Can you work these out from the model? Positions are in its coordinate system, mm. A direction names the side the tool comes from. Coordinates: 2 decimals unless noted, no trailing zeros. Order: outer loops, then holes, each group sorted by start corner. A loop starts at its lowest first (then second) coordinate and runs counter-clockwise, first axis right, second up. Notation, with made-up numbers: (5, -16.5) -> (40, -16.5) arc R18 ccw to (40, -12.5) -> close; hole circle Ø2 at (-29, 74). An arc over 180 degrees is marked (long way). Use a Markdown table: item, result. Add a question column.
1. For pin 1 Ø3.5 at (x, z) = (22.5, 19.5) entering from +Y; pin 2 Ø1.1 at (y, z) = (23, 19.5) entering from -X; pin 3 Ø4 at (x, z) = (18, 23) entering from +Y; pin 4 Ø6.5 at (y, z) = (-14.5, 16) entering from -X, each with a flat end and sliding along its axis, tell me the tip position at first contact or that it passes through.
2. If I drill on line 1 along X through (y, z) = (-5, 29.5); line 2 along Y through (x, z) = (19, 17), over which ranges is the centre line in solid material (lowest first)? Write a range as from..to.
3. Suppose I cut it at A-A, the plane z = 12. List the corners of the cut face in (x, y) for me.
4. For faces 1 (the flat face through (21.89, -0.43, 15.84)), 2 (the flat face through (-11, 17.02, 17)), 3 (the flat face through (10, 10, 13.8)), 4 (the flat face through (23, -17.02, 17)), 5 (the flat face through (23, 17.061, 17)), which set-ups out of +Z, -Z, +X, -X, +Y, -Y let a thin tool reach every point of the face, with its end or its side?
5. We'd pull the mould along Y, two halves only. Please class faces 6 (the flat face through (0, 24.9, 17)), 7 (the flat face through (19.17, -19.12, 16.66)), 8 (the flat face through (21.015, -5.842, 17.088)), 9 (the flat face through (17.061, 23, 17)): pulls with the +Y half, pulls with the -Y half, needs draft (parallel to the pull), parting line crosses it, or undercut.
6. Suppose I cut it at B-B, the plane y = -15. List the corners of the cut face in (x, z) for me.
Autodesk Inventor part; units mm, degrees
ref_plane "YZ Plane" through (0, 0, 0) normal (1, 0, 0) x (0, 1, 0)
ref_plane "XZ Plane" through (0, 0, 0) normal (0, 1, 0) x (-1, 0, 0)
ref_plane "XY Plane" through (0, 0, 0) normal (0, 0, 1) x (1, 0, 0)
ref_plane "Arbeitsebene1" through (0, 0, 0) normal (0, 0, 1) x (1, 0, 0)
sketch "Skizze1" plane through (0, 0, 0) normal (0, 0, 1) x (1, 0, 0)
  arc A0 (24.9, 22.9) -> (22.9, 24.9) centre (22.9, 22.9) ccw
  line L0 (22.9, 24.9) -> (-17.02, 24.9)
  line L1 (-17.02, 24.9) -> (-17.02, 21.2686)
  line L2 (-17.02, 21.2) -> (17.02, 21.2)
  line L3 (-21.2698, 17.02) -> (-17.02, 17.02)
  line L4 (21.2698, 17.02) -> (21.2698, -17.02)
  line L5 (21.2698, -17.02) -> (17.02, -17.02)
  line L6 (24.9, -17.02) -> (24.9, 22.9)
  line L7 (23.75, 23.25) -> (23.75, 18.15)
  arc A1 (23.25, 17.65) -> (23.75, 18.15) centre (23.25, 18.15) ccw
  line L8 (23.25, 17.65) -> (20.8937, 17.65)
  arc A2 (20.5239, 17.8134) -> (20.8937, 17.65) centre (20.8937, 18.15) ccw
  line L9 (20.5239, 17.8134) -> (17.7803, 20.8273)
  arc A3 (17.65, 21.1639) -> (17.7803, 20.8273) centre (18.15, 21.1639) ccw
  line L10 (17.65, 21.1639) -> (17.65, 23.25)
  arc A4 (18.15, 23.75) -> (17.65, 23.25) centre (18.15, 23.25) ccw
  line L11 (18.15, 23.75) -> (23.25, 23.75)
  arc A5 (23.75, 23.25) -> (23.25, 23.75) centre (23.25, 23.25) ccw
  line L12 (-17.02, 24.9) -> (17.0606, 24.9)
  line L13 (17.0606, 24.9) -> (17.0606, 21.9)
  line L14 (17.0606, 21.9) -> (-17.02, 21.9)
  line L15 (34.79, 34.79) -> (-34.79, -34.79)
  line L16 (17.0606, 21.9) -> (17.0606, 17.0606)
  line L17 (13.0606, 21.9) -> (13.0606, 13.0606)
  line L18 (17.0606, 17.0606) -> (13.0606, 13.0606)
  line L19 (17.02, 17.02) -> (-17.02, 17.02)
  line L20 (17.02, 21.2) -> (17.02, 17.02)
  line L21 (-17.02, 21.2) -> (17.02, 21.2)
  line L22 (-17.02, 24.9) -> (-17.02, 21.2686)
  line L23 (-21.2711, 17.02) -> (-17.02, 21.2686)
  line L24 (17.02, 17.02) -> (21.2698, 17.02)
  line L25 (-17.02, 21.9) -> (-13.02, 21.9)
  line L26 (-13.02, 21.9) -> (-13.02, 17.02)
  line L27 (-13.02, 17.02) -> (-17.02, 17.02)
  line L28 (-17.02, 17.02) -> (-17.02, 21.9)
  line L29 (-17.02, 21.2686) -> (-21.2711, 17.02)
  line L30 (-21.2711, 17.02) -> (-17.02, 17.02)
  line L31 (-4.9294, 21.9) -> (21.2698, -4.2993)
  line L32 (21.2698, 2.7718) -> (2.1416, 21.9)
  line L33 (12.0208, 12.0208) -> (8.4853, 8.4853)
  line L34 (-17.02, 17.02) -> (-17.02, 21.2)
  line L35 (-17.02, -21.2) -> (-17.02, -17.02)
  line L36 (-21.2698, -17.02) -> (-21.2698, 17.02)
  line L37 (-17.02, 17.02) -> (-17.02, 21.2)
  line L38 (17.02, 21.2) -> (17.02, 17.02)
  line L39 (17.02, 17.02) -> (21.2698, 17.02)
  line L40 (17.02, -17.02) -> (17.02, -21.2)
  line L41 (17.02, -21.2) -> (-17.02, -21.2)
  line L42 (-20.8273, -17.7803) -> (-17.8134, -20.5239)
  arc A6 (-17.65, -20.8937) -> (-17.8134, -20.5239) centre (-18.15, -20.8937) ccw
  line L43 (-17.65, -20.8937) -> (-17.65, -23.25)
  arc A7 (-18.15, -23.75) -> (-17.65, -23.25) centre (-18.15, -23.25) ccw
  line L44 (-18.15, -23.75) -> (-23.25, -23.75)
  arc A8 (-23.75, -23.25) -> (-23.25, -23.75) centre (-23.25, -23.25) ccw
  line L45 (-23.75, -23.25) -> (-23.75, -18.15)
  arc A9 (-23.25, -17.65) -> (-23.75, -18.15) centre (-23.25, -18.15) ccw
  line L46 (-23.25, -17.65) -> (-21.1639, -17.65)
  arc A10 (-20.8273, -17.7803) -> (-21.1639, -17.65) centre (-21.1639, -18.15) ccw
  line L47 (-21.2711, 17.02) -> (-17.02, 21.2686)
  line L48 (-21.2711, 17.02) -> (-24.9, 17.02)
  line L49 (-24.9, 17.02) -> (-24.9, -22.9)
  arc A11 (-24.9, -22.9) -> (-22.9, -24.9) centre (-22.9, -22.9) ccw
  line L50 (-22.9, -24.9) -> (17.02, -24.9)
  line L51 (17.02, -24.9) -> (17.02, -21.2686)
  line L52 (21.2711, -17.02) -> (17.02, -21.2686)
  line L53 (21.2711, -17.02) -> (24.9, -17.02)
  line L54 (-17.02, -21.2) -> (-17.02, -17.02)
  line L55 (-17.02, -17.02) -> (-21.2698, -17.02)
  line L56 (-21.2698, -17.02) -> (-21.2698, 17.02)
  line L57 (-17.02, 17.02) -> (-17.02, 21.2)
  line L58 (-17.02, 21.2) -> (17.02, 21.2)
  line L59 (17.02, 21.2) -> (17.02, 17.02)
  line L60 (21.2698, 17.02) -> (21.2698, -17.02)
  line L61 (21.2698, -17.02) -> (17.02, -17.02)
  line L62 (17.02, -17.02) -> (17.02, -21.2)
  line L63 (17.02, -21.2) -> (-17.02, -21.2)
  line L64 (-20.8273, -17.7803) -> (-17.8134, -20.5239)
  arc A12 (-17.65, -20.8937) -> (-17.8134, -20.5239) centre (-18.15, -20.8937) ccw
  line L65 (-17.65, -20.8937) -> (-17.65, -23.25)
  arc A13 (-18.15, -23.75) -> (-17.65, -23.25) centre (-18.15, -23.25) ccw
  line L66 (-18.15, -23.75) -> (-23.25, -23.75)
  arc A14 (-23.75, -23.25) -> (-23.25, -23.75) centre (-23.25, -23.25) ccw
  line L67 (-23.75, -23.25) -> (-23.75, -18.15)
  arc A15 (-23.25, -17.65) -> (-23.75, -18.15) centre (-23.25, -18.15) ccw
  line L68 (-23.25, -17.65) -> (-21.1639, -17.65)
  arc A16 (-20.8273, -17.7803) -> (-21.1639, -17.65) centre (-21.1639, -18.15) ccw
  line L69 (23.75, 23.25) -> (23.75, 18.15)
  arc A17 (23.25, 17.65) -> (23.75, 18.15) centre (23.25, 18.15) ccw
  line L70 (23.25, 17.65) -> (20.8937, 17.65)
  arc A18 (20.5239, 17.8134) -> (20.8937, 17.65) centre (20.8937, 18.15) ccw
  line L71 (20.5239, 17.8134) -> (17.7803, 20.8273)
  arc A19 (17.65, 21.1639) -> (17.7803, 20.8273) centre (18.15, 21.1639) ccw
  line L72 (17.65, 21.1639) -> (17.65, 23.25)
  arc A20 (18.15, 23.75) -> (17.65, 23.25) centre (18.15, 23.25) ccw
  line L73 (18.15, 23.75) -> (23.25, 23.75)
  arc A21 (23.75, 23.25) -> (23.25, 23.75) centre (23.25, 23.25) ccw
  arc A22 (24.9, 22.9) -> (22.9, 24.9) centre (22.9, 22.9) ccw
  line L74 (22.9, 24.9) -> (-17.02, 24.9)
  line L75 (-21.2711, 17.02) -> (-24.9, 17.02)
  line L76 (-24.9, 17.02) -> (-24.9, -22.9)
  arc A23 (-24.9, -22.9) -> (-22.9, -24.9) centre (-22.9, -22.9) ccw
  line L77 (-22.9, -24.9) -> (17.02, -24.9)
  line L78 (17.02, -24.9) -> (17.02, -21.2686)
  line L79 (21.2711, -17.02) -> (17.02, -21.2686)
  line L80 (21.2711, -17.02) -> (24.9, -17.02)
  line L81 (24.9, -17.02) -> (24.9, 22.9)
  line L82 (19.2323, 19.2323) -> (17.0606, 21.6178)
  line L83 (-17.02, -17.02) -> (-21.2698, -17.02)
  line L84 (-21.2698, 17.02) -> (-17.02, 17.02)
  point P0 (0, 0)
  point P1 (17.0606, 24.9)
  point P2 (-16.97, 16.97)
  point P3 (-13.02, 17.02)
  point P4 (-13.02, 21.2)
  point P5 (13.0606, 21.2)
  point P6 (2.8416, 21.2)
  point P7 (-4.2294, 21.2)
  point P8 (13.0606, 17.02)
  point P9 (16.97, 21.2)
  point P10 (-16.97, 17.02)
  point P11 (-17.02, 20.7)
  point P12 (13.0606, 21.2)
  point P13 (-16.97, 21.2)
  point P14 (-17.02, 21.9)
  point P15 (19.2323, 19.2323)
  point P16 (23.6036, 23.6036)
  point P17 (24.3142, 24.3142)
  point P18 (16.97, 17.02)
  point P19 (7.0216, 17.02)
  point P20 (-0.0494, 17.02)
  point P21 (-17.02, 17.02)
  dimension "d3" = 4
  dimension "d6" = 4
  dimension "d9" = 0
  dimension "d11" = 5
  dimension "d35" = 0
extrude "Extrusion1" add sketch "Skizze1" along normal blind 33.8 contours L13 L14 L1 L0 | L15 L16 L82 L9 | L16 L15 L20 L2 L17 L14 | L31 L19 L32 L15 | L14 L26 L2 L28 L1 | L17 L2 L32 L14 | L15 L17 L19 | L19 L17 L2 L20 | L32 L19 L17 L15 | L31 L2 L32 L19 | L19 L26 L2 L31 | L28 L3 L23 | L14 L31 L2 L26 | L32 L2 L31 L14 | L17 L19 L32 L2 | L19 L28 L2 L26
mirror "Spiegeln1" about plane through (8.4853, 8.4853, 0) normal (0.7071, -0.7071, 0) of "Extrusion1"
sketch "Skizze2" plane through (17.6463, 20.9745, 0) normal (0.7395, 0.6732, 0) x (-0.6732, 0.7395, 0)
  circle A0 centre (-16.6729, 31.13) radius 1.45
  circle A1 centre (-16.6729, 3.13) radius 1.45
  circle A2 centre (11.3271, 31.13) radius 1.45
  point P0 (-3.6312, 0)
  dimension "d36" = 2.9
  dimension "d37" = 2.9
  dimension "d38" = 2.9
sketch "Skizze3" plane through (17.2397, 21.0462, 0) normal (0.6732, 0.7395, 0) x (-0.7395, 0.6732, 0)
  line L0 (-17.8955, 20.13) -> (-17.8955, 14.13)
  line L1 (-20.8922, 14.13) -> (-20.8922, 20.13)
  line L2 (-0.9142, 31.21) -> (-6.9076, 31.21)
  line L3 (-6.9076, 34.21) -> (-0.9142, 34.21)
  line L4 (13.0291, 42.03) -> (-20.8922, 42.03)
  line L5 (-20.8922, 42.03) -> (-20.8922, 38.4552)
  line L6 (-20.8922, 38.4552) -> (-25.2126, 34.13)
  line L7 (-25.2126, 34.13) -> (-28.7835, 34.13)
  line L8 (-28.7835, 34.13) -> (-28.7835, 0.13)
  line L9 (-28.7835, 0.13) -> (-25.2126, 0.13)
  line L10 (-25.2126, 0.13) -> (-20.8922, -4.1952)
  line L11 (-20.8922, -4.1952) -> (-20.8922, -7.77)
  line L12 (-20.8922, -7.77) -> (13.0704, -7.77)
  line L13 (13.0704, -7.77) -> (13.0704, -4.1952)
  line L14 (13.0704, -4.1952) -> (17.3909, 0.13)
  line L15 (17.3909, 0.13) -> (20.9618, 0.13)
  line L16 (20.9618, 0.13) -> (20.9618, 34.13)
  line L17 (20.9618, 34.13) -> (17.3909, 34.13)
  line L18 (17.3909, 34.13) -> (13.0291, 38.4966)
  line L19 (13.0291, 38.4966) -> (13.0291, 42.03)
  ellipse E0 centre (-19.3938, 14.13) end of major axis (-19.3938, 15.63) minor radius 1.4984 (-20.8922, 14.13) -> (-17.8955, 14.13) ccw
  ellipse E1 centre (-19.3938, 20.13) end of major axis (-19.3938, 18.63) minor radius 1.4984 (-17.8955, 20.13) -> (-20.8922, 20.13) ccw
  ellipse E2 centre (-6.9076, 32.71) end of major axis (-6.9076, 34.21) minor radius 1.4984 (-6.9076, 34.21) -> (-6.9076, 31.21) ccw
  ellipse E3 centre (-0.9142, 32.71) end of major axis (-0.9142, 31.21) minor radius 1.4984 (-0.9142, 31.21) -> (-0.9142, 34.21) ccw
  ellipse E4 centre (-17.8955, 31.13) end of major axis (-17.8955, 34.38) minor radius 3.2464
  ellipse E5 centre (-3.9109, 17.13) end of major axis (-3.9109, 20.38) minor radius 3.2464
  ellipse E6 centre (10.0737, 31.13) end of major axis (10.0737, 34.38) minor radius 3.2464
  ellipse E7 centre (-17.8955, 3.13) end of major axis (-17.8955, 6.38) minor radius 3.2464
  point P0 (-1.4194, 0)
extrude "Extrusion2" cut sketch "Skizze3" against normal blind 33.8 contours L0 E0 L1 E1 | L2 E2 L3 E3
sketch "Skizze4" plane through (0, 0, 33.8) normal (0, 0, 1) x (1, 0, 0)
  line L0 (22.3477, 16.3962) -> (11.972, 4.9986)
  line L1 (17.9157, 20.4308) -> (7.7294, 9.2412)
  circle A0 centre (10.3701, 10.3701) radius 1.4
  line L2 (19.2323, 19.2323) -> (21.6178, 17.0606)
  line L3 (19.2323, 19.2323) -> (17.9157, 20.4308)
  line L4 (11.972, 4.9986) -> (7.7294, 9.2412)
  line L5 (22.3477, 16.3962) -> (21.6178, 17.0606)
  point P0 (0, 0)
  dimension "d26" = 2.8
extrude "Extrusion3" cut sketch "Skizze4" against normal blind 20 contours A0 L1 | L1 A0
sketch "Skizze5" plane through (24.9, -16.97, 33.8) normal (1, 0, 0) x (0, 0, -1)
  line L0 (0, 34.0306) -> (0, -0.05)
  line L1 (33.8, 34.0306) -> (33.8, -0.05)
  line L2 (19.67, 15.5558) -> (13.67, 15.5558)
  circle A0 centre (16.67, 15.5558) radius 1.4
  line L3 (33.8, -0.05) -> (0, -0.05)
  line L4 (33.8, 34.0306) -> (0, 34.0306)
  point P0 (33.8, 16.97)
  dimension "d29" = 2.8
extrude "Extrusion4" cut sketch "Skizze5" against normal blind 20 contours A0 L2 | L2 A0
extrude "Extrusion6" cut sketch "Skizze2" against normal through all
properties part number "20_Cube_Insert_Kinematic_Mirror_45_pro_v3"
Worked out:
| question | item | result |
|---|---|---|
| 1 | pin 1 | stops at y = 17.85 |
| 1 | pin 2 | stops at x = -17.02 |
| 1 | pin 3 | stops at y = 24.9 |
| 1 | pin 4 | stops at x = 17.02 |
| 2 | line 1 | x = 17.02..24.9 |
| 2 | line 2 | y = -19.29..-8.06, -3.6..-2.81, -0.02..19.49 |
| 3 | outline | (-21.27, 17.02) -> (-0.05, 17.02) -> (8.49, 8.49) -> (17.02, -0.05) -> (17.02, -21.27) -> (21.27, -17.02) -> (24.9, -17.02) -> (24.9, 17.06) -> (21.62, 17.06) -> (20.83, 17.78) -> (19.23, 19.23) -> (17.78, 20.83) -> (17.06, 21.62) -> (17.06, 24.9) -> (-17.02, 24.9) -> (-17.02, 21.27) -> close |
| 4 | face 1 | none |
| 4 | face 2 | +Z, -Z, -X, -Y |
| 4 | face 3 | +Z |
| 4 | face 4 | +Z, -Z, +X, -Y |
| 4 | face 5 | +Z, -Z, +X, +Y |
| 5 | face 6 | pulls with the +Y half |
| 5 | face 7 | pulls with the -Y half |
| 5 | face 8 | undercut |
| 5 | face 9 | needs draft |
| 6 | outline | (17.02, 0) -> (24.9, 0) -> (24.9, 33.8) -> (17.02, 33.8) -> close |
